Design review of the part built by this model. Coordinates are the model's own, in mm. A direction names the side the tool comes from. Coordinates: 2 decimals unless noted, no trailing zeros. Write each loop counter-clockwise with the first axis right and the second up, starting at its lowest first coordinate (ties: lowest second). Pieces come first, ordered by that corner, then holes. Notation, with made-up numbers: (-24.75, 53.25) - (30.25, 53.25) arc R8 ccw to (30.25, 64.25) - close; hole circle Ø6 at (73, 86.5). An arc over 180 degrees is marked (long way). Answer as a JSON object with one key per item and string values.
```python
from build123d import *

# Parameters (mm, degrees)
BOSS_EXTRUDE1_DEPTH = 12.7
SKETCH2_R           = 3.175
CUT_EXTRUDE1_DEPTH  = 13.7


with BuildPart() as part:
    # Sketch1 → Boss-Extrude1 (new body)
    with BuildSketch(Plane(origin=(0, 0, 0), x_dir=(1, 0, 0), z_dir=(0, 1, 0))):
        with BuildLine():
            Line((0, 0), (-12.7, 0))
            Line((-12.7, 0), (-12.7, -4.7625))
            Line((-12.7, -4.7625), (-2.749630657, -4.7625))
            ThreePointArc((-2.749630657, -4.7625), (3.175, -6.35), (-2.749630657, -7.9375))
            Line((-2.749630657, -7.9375), (-12.7, -7.9375))
            Line((-12.7, -7.9375), (-12.7, -12.7))
            Line((-12.7, -12.7), (0, -12.7))
            ThreePointArc((0, -12.7), (6.35, -6.35), (0, 0))
        make_face()
    extrude(amount=BOSS_EXTRUDE1_DEPTH)

    # Sketch2 → Cut-Extrude1 (cut, through all)
    with BuildSketch(Plane.XY.offset(12.7)):
        with Locations((-6.35, 6.35)):
            Circle(SKETCH2_R)
    extrude(amount=-CUT_EXTRUDE1_DEPTH, mode=Mode.SUBTRACT)


solid = part.part
```
(1) To check wall thickness, follow line 1 (Y direction, x = -6.35, z = 11.7) (3 decimals); line 2 (Z direction, x = -10.5, y = 1); line 3 (X direction, y = 8.5, z = 6.35) (3 decimals). State the ranges of each line that lie inside material, in increasing order. Write a range as from..to.
Solved:
{"line 1": "y = 0..3.175, 9.525..12.7", "line 2": "z = 0..4.76, 7.94..12.7", "line 3": "x = 3.175..6.35"}
(2) Take a section at B-B, the plane x = -6.35. Write out the cut boundary in (y, z) (1 decimal), and give its area (3 significant figures).
Solved:
{"outline": "(0, 0) - (3.2, 0) - (3.2, 4.8) - (0, 4.8) - close; (0, 7.9) - (3.2, 7.9) - (3.2, 12.7) - (0, 12.7) - close; (9.5, 0) - (12.7, 0) - (12.7, 4.8) - (9.5, 4.8) - close; (9.5, 7.9) - (12.7, 7.9) - (12.7, 12.7) - (9.5, 12.7) - close", "area": "60.5 mm^2"}
(3) The part is to be moulded in two halves that separate along Z. For faces 1 (the face through (6.35, 6.26, 6.49)), 2 (the face through (-3, 0, 9)), 3 (the face through (-8, 3, 12.7)), 4 (the face through (-10, 6, 4.762)), say which applies: pulls with the +Z half, pulls with the -Z half, needs draft (parallel to the pull), parting line crosses it, or undercut.
Solved:
{"face 1": "parting line crosses it", "face 2": "needs draft", "face 3": "pulls with the +Z half", "face 4": "undercut"}
(4) For pin 1 (3 mm diameter, centred on y = 7, z = 10.5, fed in from +X); pin 2 (2 mm diameter, centred on x = 2, y = 10.5, fed in from -Z), all flat-tipped, find the tip position at first contact; note any pin that passes through.
Solved:
{"pin 1": "stops at x = 5.77", "pin 2": "stops at z = 0.08"}
(5) Take a section at D-D, the plane z = 1.5. Write out the cut boundary in (x, y) (3 decimals).
Solved:
{"outline": "(-12.7, 0) - (4.099, 0) - (4.099, 12.7) - (-12.7, 12.7) - close; hole circle Ø6.35 at (-6.35, 6.35)"}
(6) Tool access review of faces 5 (the face through (-10, 6, 7.938)), 6 (the face through (-12.7, 6, 2)): name each direction out of +Z, -Z, +X, -X, +Y, -Y from which nothing blocks a thin tool from reaching the whole face with its end or side.
Solved:
{"face 5": "-X, +Y, -Y", "face 6": "+Z, -Z, -X, +Y, -Y"}
(7) Take a section at C-C, the plane x = -1.75. Write out the cut boundary in (y, z), and give its area (3 significant figures).
Solved:
{"outline": "(0, 0) - (12.7, 0) - (12.7, 3.7) - (0, 3.7) - close; (0, 9) - (12.7, 9) - (12.7, 12.7) - (0, 12.7) - close", "area": "94.0 mm^2"}
(8) Take a section at A-A, the plane y = 6.35. Give the number of separate pieces and of enclosed holes in the cut face, and give its area (3 significant figures).
Solved:
{"separate pieces": "3", "enclosed holes": "0", "area": "102 mm^2"}
